Verification items for the finished model (mm, model axes). A direction names the side the tool comes from. Give positions to 0.01 mm unless a question says otherwise; leave off trailing zeros. Write each loop counter-clockwise with the first axis right and the second up, starting at its lowest first coordinate (ties: lowest second). Pieces come first, ordered by that corner, then holes. Notation, with made-up numbers: (-38.75, 45.5) -> (-25.75, 45.5) arc R30 cw to (-25.75, 74.5) -> close; hole circle Ø4 at (4, 29.25). An arc over 180 degrees is marked (long way). Use one line per item in the form item = value. Start each with the question number.
(1) Section check B-B, the plane y = -6. Record the cut outline in (x, z).
(2) Section check D-D, the plane x = -25. Record the cut outline in (y, z).
(3) Set-up check for faces 5 (the face through (0, 2.1, 5)), 6 (the face through (-55.07, -14.297, 63.986)), 7 (the face through (-45, 0, 15)), 8 (the face through (1.4, 10.6, 6.6)): record each of +Z, -Z, +X, -X, +Y, -Y from which the full face is reachable in a straight line by a thin tool's end or side.
(4) Section check A-A, the plane z = 53. Record the cut outline in (x, y), plus the area to 3 significant figures.
(5) Scan lines: L1, parallel to Y at x = 0, z = 7.9; L2, parallel to X at y = -5, z = 55.5; L3, parallel to X at y = -14, z = 13. Record each from-to range of solid material in increasing order.
(6) Release check for a two-part mould opening along X. For faces 1 (the face through (7.145, -5.857, 8.324)), 2 (the face through (55, 0, 5)), 3 (the face through (-12.09, -5.93, 3.35)), 4 (the face through (-60, 0, 40)) record: pulls with the +X half, pulls with the -X half, needs draft (parallel to the pull), parting line crosses it, or undercut.
(7) Depth check by flat-ended pin: pin 1 Ø10.5 at (x, y) = (-10.39, -6) entering from +Z; pin 2 Ø3 at (y, z) = (-11.5, 9) entering from -X; pin 3 Ø5.5 at (x, y) = (0, 12) entering from +Z; pin 4 Ø2 at (x, y) = (-10.39, -6) entering from +Z. Enter the tip coordinate at first touch or a pass-through.
(8) Section check C-C, the plane y = 12. Record the cut outline in (x, z).
from build123d import *

# Parameters (mm, degrees)
AUFSATZ_LINEAR_AUSTRAGEN1_DEPTH = 20
SCHNITT_LINEAR_AUSTRAGEN1_DEPTH = 20
FASE1_SIZE                      = 10
VERRUNDUNG1_R                   = 20
SKIZZE3_R                       = 3.25
SCHNITT_LINEAR_AUSTRAGEN2_DEPTH = 3.4
SKIZZE4_R                       = 1.7
SCHNITT_LINEAR_AUSTRAGEN3_DEPTH = 6.6
KREISMUSTER1_COUNT              = 3


with BuildPart() as part:
    # Skizze1 → Aufsatz-Linear austragen1 (new, symmetric)
    with BuildSketch(Plane(origin=(0, 0, 0), x_dir=(1, 0, 0), z_dir=(0, 1, 0))):
        Polygon((-60, 0), (60, 0), (60, -70), (50, -70), (50, -10), (-50, -10), (-50, -70), (-60, -70), align=None)
    extrude(amount=AUFSATZ_LINEAR_AUSTRAGEN1_DEPTH, both=True)

    # Skizze2 → Schnitt-Linear austragen1 (cut)
    with BuildSketch(Plane(origin=(0, 0, 0), x_dir=(-1, 0, 0), z_dir=(0, 0, -1))):
        with BuildLine():
            Line((-1.532970972, 2.1), (1.532970972, 2.1))
            ThreePointArc((1.532970972, 2.1), (0, -2.6), (-1.532970972, 2.1))
        make_face()
    extrude(amount=-SCHNITT_LINEAR_AUSTRAGEN1_DEPTH, mode=Mode.SUBTRACT)

    # Fase1
    fase1_edges = [part.edges().sort_by_distance(p)[0] for p in [
        (-60, 0, 0),
        (60, 0, 0),
        (50, 0, 10),
        (-50, 0, 10),
    ]]
    chamfer(fase1_edges, length=FASE1_SIZE)

    # Verrundung1
    verrundung1_edges = [part.edges().sort_by_distance(p)[0] for p in [
        (-55, -20, 70),
        (-55, 20, 70),
        (55, 20, 70),
        (55, -20, 70),
    ]]
    fillet(verrundung1_edges, radius=VERRUNDUNG1_R - 0.0001)  # a hair under: the kernel refuses the full size

    # Skizze3 → Schnitt-Linear austragen2 (cut)
    with BuildSketch(Plane.XY.offset(10)):
        with Locations((0, 12)):
            Circle(SKIZZE3_R)
    schnitt_linear_austragen2 = extrude(amount=-SCHNITT_LINEAR_AUSTRAGEN2_DEPTH, mode=Mode.SUBTRACT)

    # Skizze4 → Schnitt-Linear austragen3 (cut)
    with BuildSketch(Plane.XY.offset(6.6)):
        with Locations((0, 12)):
            Circle(SKIZZE4_R)
    schnitt_linear_austragen3 = extrude(amount=-SCHNITT_LINEAR_AUSTRAGEN3_DEPTH, mode=Mode.SUBTRACT)

    # Kreismuster1: Schnitt-Linear austragen2, Schnitt-Linear austragen3 ×3 about axis
    kreismuster1_axis = Axis((0, 0, 0), (0, 0, 1))
    add([schnitt_linear_austragen2.rotate(kreismuster1_axis, i * 360 / KREISMUSTER1_COUNT) for i in range(1, KREISMUSTER1_COUNT)], mode=Mode.SUBTRACT)
    add([schnitt_linear_austragen3.rotate(kreismuster1_axis, i * 360 / KREISMUSTER1_COUNT) for i in range(1, KREISMUSTER1_COUNT)], mode=Mode.SUBTRACT)


solid = part.part
Completed:
q1.outline = (-60, 10) -> (-50, 0) -> (-12.09, 0) -> (-12.09, 6.6) -> (-13.64, 6.6) -> (-13.64, 10) -> (-40, 10) -> (-50, 20) -> (-50, 69.08) -> (-60, 69.08) -> close; (-8.69, 0) -> (8.69, 0) -> (8.69, 6.6) -> (7.14, 6.6) -> (7.14, 10) -> (-7.14, 10) -> (-7.14, 6.6) -> (-8.69, 6.6) -> close; (12.09, 0) -> (50, 0) -> (60, 10) -> (60, 69.08) -> (50, 69.08) -> (50, 20) -> (40, 10) -> (13.64, 10) -> (13.64, 6.6) -> (12.09, 6.6) -> close
q2.outline = (-20, 0) -> (20, 0) -> (20, 10) -> (-20, 10) -> close
q3.face_5 = +Z, -Z
q3.face_6 = +Z, +X, -X, -Y
q3.face_7 = +Z, +Y, -Y
q3.face_8 = +Z
q4.outline = (-60, -19.77) -> (-50, -19.77) -> (-50, 19.77) -> (-60, 19.77) -> close; (50, -19.77) -> (60, -19.77) -> (60, 19.77) -> (50, 19.77) -> close
q4.area = 791 mm²
q5.L1 = -20 to -2.6, 2.1 to 8.75, 15.25 to 20
q5.L2 = -60 to -50, 50 to 60
q5.L3 = -60 to -43, 43 to 60
q6.face_1 = undercut
q6.face_2 = pulls with the +X half
q6.face_3 = undercut
q6.face_4 = pulls with the -X half
q7.pin_1 = 10
q7.pin_2 = -60
q7.pin_3 = 6.6
q7.pin_4 = through
q8.outline = (-60, 10) -> (-50, 0) -> (-1.7, 0) -> (-1.7, 6.6) -> (-3.25, 6.6) -> (-3.25, 10) -> (-40, 10) -> (-50, 20) -> (-50, 66) -> (-60, 66) -> close; (1.7, 0) -> (50, 0) -> (60, 10) -> (60, 66) -> (50, 66) -> (50, 20) -> (40, 10) -> (3.25, 10) -> (3.25, 6.6) -> (1.7, 6.6) -> close
